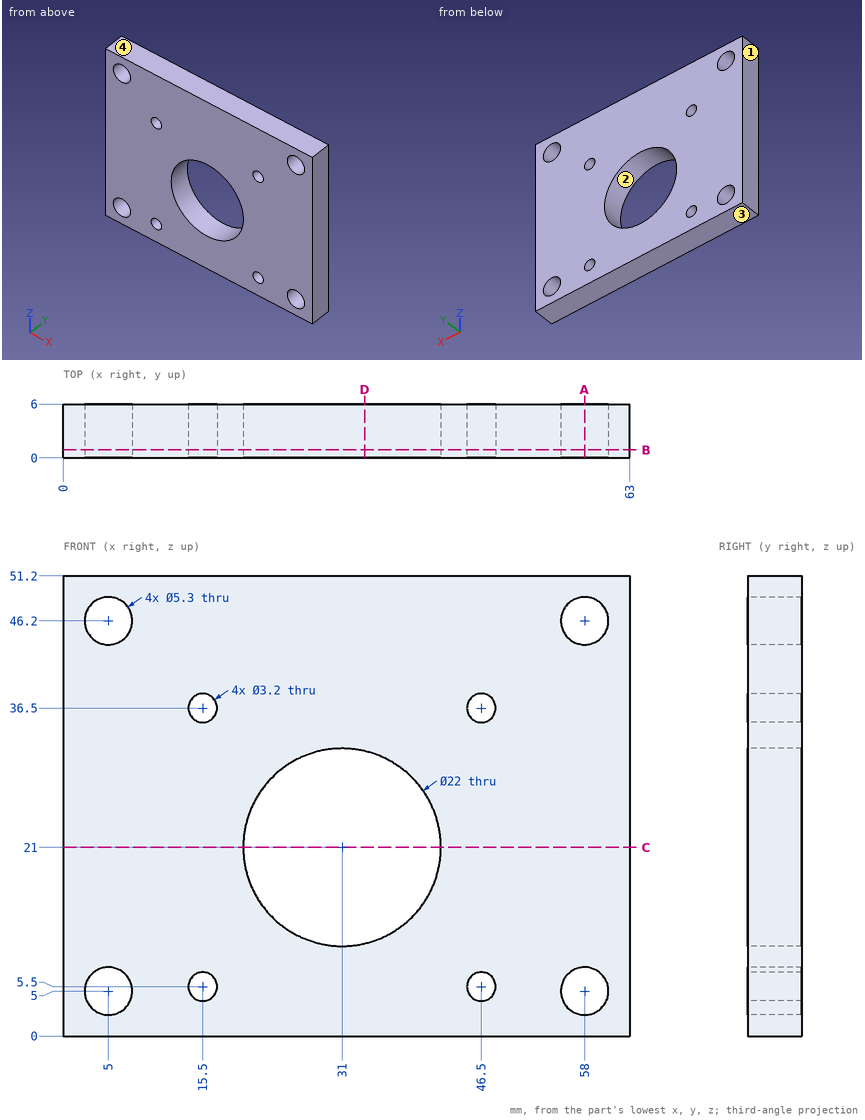
Geometry: see drawing. Coordinates: mm, zero at the bounding-box minimum. Give positions to 0.01 mm unless a question says otherwise; leave off trailing zeros. Loops run counter-clockwise (first coordinate to the right, second up) from the corner with the lowest first, then second, coordinate; pieces in that order, holes last. Notation, with made-up numbers: M 13.5,45 L 57.5,45 A25 cw 57.5,65 Z; hole C 55.5,41.25 d3. An arc over 180 degrees is marked long. Use one line per item in the form item = value.
1. Section query C-C, the plane z = 21. Return the cut outline in (x, y).
Numbers:
outline = M 0,0 L 20,0 L 20,6 L 0,6 Z; M 42,0 L 63,0 L 63,6 L 42,6 Z
2. Section query B-B, the plane y = 0.9. Count the separate pieces of the cut face and the enclosed holes in it, and give its area (3 significant figures).
Numbers:
separate_pieces = 1
enclosed_holes = 9
area = 2,730 mm²
3. Section query D-D, the plane x = 33.5. Return the cut outline in (y, z).
Numbers:
outline = M 0,0 L 6,0 L 6,10.29 L 0,10.29 Z; M 0,31.71 L 6,31.71 L 6,51.2 L 0,51.2 Z
4. Pull-direction query (Z, two-part tool) for the marked faces 1, 2, 3 and 4; classes: released by +Z, released by -Z, zero draft, split by the parting line, or undercut.
Numbers:
face_1 = zero draft
face_2 = undercut
face_3 = released by -Z
face_4 = released by +Z
5. Section query A-A, the plane x = 58. Return the cut outline in (y, z), and give its area (3 significant figures).
Numbers:
outline = M 0,0 L 6,0 L 6,2.35 L 0,2.35 Z; M 0,7.65 L 6,7.65 L 6,43.55 L 0,43.55 Z; M 0,48.85 L 6,48.85 L 6,51.2 L 0,51.2 Z
area = 244 mm²
6. Line query: L1, parallel to Z at x = 58, y = 3.6; L2, parallel to Z at x = 46.5, y = 3.2; L3, parallel to X at y = 2, z = 46.2. Output: solid intervals per line, ascending.
Numbers:
L1 = 0 to 2.35, 7.65 to 43.55, 48.85 to 51.2
L2 = 0 to 3.9, 7.1 to 34.9, 38.1 to 51.2
L3 = 0 to 2.35, 7.65 to 55.35, 60.65 to 63
